from build123d import *

# Parameters (mm, degrees)
F2_DEPTH = 10


with BuildPart() as f2:
    # F1 (on Front) → F2 (new body)
    with BuildSketch(Plane.XZ):
        with BuildLine():
            Line((3.4480698746, 29.0000970366), (1.2642837874, 35))
            Line((1.2642837874, 35), (-1.2642837874, 35))
            Line((-1.2642837874, 35), (-3.4480698746, 29.0000970366))
            ThreePointArc((-3.4480698746, 29.0000970366), (-3.8654423248, 28.4561666695), (-4.5193194622, 28.25))
            Line((-4.5193194622, 28.25), (-4.7123889804, 28.25))
            Line((-4.7123889804, 28.25), (-4.7123889804, 0))
            Line((-4.7123889804, 0), (4.7123889804, 0))
            Line((4.7123889804, 0), (4.7123889804, 28.25))
            Line((4.7123889804, 28.25), (4.5193194622, 28.25))
            ThreePointArc((4.5193194622, 28.25), (3.8654423248, 28.4561666695), (3.4480698746, 29.0000970366))
        make_face()
        with BuildLine():
            Line((4.9054584985, 28.25), (4.7123889804, 28.25))
            Line((4.7123889804, 28.25), (4.7123889804, 0))
            Line((4.7123889804, 0), (14.1371669412, 0))
            Line((14.1371669412, 0), (14.1371669412, 28.25))
            Line((14.1371669412, 28.25), (13.944097423, 28.25))
            ThreePointArc((13.944097423, 28.25), (13.2902202856, 28.4561666695), (12.8728478353, 29.0000970366))
            Line((12.8728478353, 29.0000970366), (10.6890617482, 35))
            Line((10.6890617482, 35), (8.1604941734, 35))
            Line((8.1604941734, 35), (5.9767080862, 29.0000970366))
            ThreePointArc((5.9767080862, 29.0000970366), (5.559335636, 28.4561666695), (4.9054584985, 28.25))
        make_face()
        with BuildLine():
            Line((14.1371669412, 28.25), (14.1371669412, 0))
            Line((14.1371669412, 0), (23.5619449019, 0))
            Line((23.5619449019, 0), (23.5619449019, 28.25))
            Line((23.5619449019, 28.25), (23.3688753838, 28.25))
            ThreePointArc((23.3688753838, 28.25), (22.7149982463, 28.4561666695), (22.2976257961, 29.0000970366))
            Line((22.2976257961, 29.0000970366), (20.1138397089, 35))
            Line((20.1138397089, 35), (17.5852721341, 35))
            Line((17.5852721341, 35), (15.401486047, 29.0000970366))
            ThreePointArc((15.401486047, 29.0000970366), (14.9841135967, 28.4561666695), (14.3302364593, 28.25))
            Line((14.3302364593, 28.25), (14.1371669412, 28.25))
        make_face()
        with BuildLine():
            Line((23.5619449019, 28.25), (23.5619449019, 0))
            Line((23.5619449019, 0), (32.9867228627, 0))
            Line((32.9867228627, 0), (32.9867228627, 28.25))
            Line((32.9867228627, 28.25), (32.7936533446, 28.25))
            ThreePointArc((32.7936533446, 28.25), (32.1397762071, 28.4561666695), (31.7224037569, 29.0000970366))
            Line((31.7224037569, 29.0000970366), (29.5386176697, 35))
            Line((29.5386176697, 35), (27.0100500949, 35))
            Line((27.0100500949, 35), (24.8262640078, 29.0000970366))
            ThreePointArc((24.8262640078, 29.0000970366), (24.4088915575, 28.4561666695), (23.7550144201, 28.25))
            Line((23.7550144201, 28.25), (23.5619449019, 28.25))
        make_face()
        with BuildLine():
            Line((32.9867228627, 28.25), (32.9867228627, 0))
            Line((32.9867228627, 0), (42.4115008235, 0))
            Line((42.4115008235, 0), (42.4115008235, 28.25))
            Line((42.4115008235, 28.25), (42.2184313053, 28.25))
            ThreePointArc((42.2184313053, 28.25), (41.5645541679, 28.4561666695), (41.1471817176, 29.0000970366))
            Line((41.1471817176, 29.0000970366), (38.9633956305, 35))
            Line((38.9633956305, 35), (36.4348280557, 35))
            Line((36.4348280557, 35), (34.2510419685, 29.0000970366))
            ThreePointArc((34.2510419685, 29.0000970366), (33.8336695183, 28.4561666695), (33.1797923808, 28.25))
            Line((33.1797923808, 28.25), (32.9867228627, 28.25))
        make_face()
        with BuildLine():
            Line((42.4115008235, 28.25), (42.4115008235, 0))
            Line((42.4115008235, 0), (51.8362787842, 0))
            Line((51.8362787842, 0), (51.8362787842, 28.25))
            Line((51.8362787842, 28.25), (51.6432092661, 28.25))
            ThreePointArc((51.6432092661, 28.25), (50.9893321287, 28.4561666695), (50.5719596784, 29.0000970366))
            Line((50.5719596784, 29.0000970366), (48.3881735912, 35))
            Line((48.3881735912, 35), (45.8596060165, 35))
            Line((45.8596060165, 35), (43.6758199293, 29.0000970366))
            ThreePointArc((43.6758199293, 29.0000970366), (43.258447479, 28.4561666695), (42.6045703416, 28.25))
            Line((42.6045703416, 28.25), (42.4115008235, 28.25))
        make_face()
        with BuildLine():
            Line((51.8362787842, 28.25), (51.8362787842, 0))
            Line((51.8362787842, 0), (61.261056745, 0))
            Line((61.261056745, 0), (61.261056745, 28.25))
            Line((61.261056745, 28.25), (61.0679872269, 28.25))
            ThreePointArc((61.0679872269, 28.25), (60.4141100894, 28.4561666695), (59.9967376392, 29.0000970366))
            Line((59.9967376392, 29.0000970366), (57.812951552, 35))
            Line((57.812951552, 35), (55.2843839772, 35))
            Line((55.2843839772, 35), (53.1005978901, 29.0000970366))
            ThreePointArc((53.1005978901, 29.0000970366), (52.6832254398, 28.4561666695), (52.0293483024, 28.25))
            Line((52.0293483024, 28.25), (51.8362787842, 28.25))
        make_face()
        with BuildLine():
            Line((61.261056745, 28.25), (61.261056745, 0))
            Line((61.261056745, 0), (70.6858347058, 0))
            Line((70.6858347058, 0), (70.6858347058, 28.25))
            Line((70.6858347058, 28.25), (70.4927651876, 28.25))
            ThreePointArc((70.4927651876, 28.25), (69.8388880502, 28.4561666695), (69.4215155999, 29.0000970366))
            Line((69.4215155999, 29.0000970366), (67.2377295128, 35))
            Line((67.2377295128, 35), (64.709161938, 35))
            Line((64.709161938, 35), (62.5253758508, 29.0000970366))
            ThreePointArc((62.5253758508, 29.0000970366), (62.1080034006, 28.4561666695), (61.4541262631, 28.25))
            Line((61.4541262631, 28.25), (61.261056745, 28.25))
        make_face()
        with BuildLine():
            Line((70.6858347058, 28.25), (70.6858347058, 0))
            Line((70.6858347058, 0), (80.1106126665, 0))
            Line((80.1106126665, 0), (80.1106126665, 28.25))
            Line((80.1106126665, 28.25), (79.9175431484, 28.25))
            ThreePointArc((79.9175431484, 28.25), (79.263666011, 28.4561666695), (78.8462935607, 29.0000970366))
            Line((78.8462935607, 29.0000970366), (76.6625074735, 35))
            Line((76.6625074735, 35), (74.1339398988, 35))
            Line((74.1339398988, 35), (71.9501538116, 29.0000970366))
            ThreePointArc((71.9501538116, 29.0000970366), (71.5327813613, 28.4561666695), (70.8789042239, 28.25))
            Line((70.8789042239, 28.25), (70.6858347058, 28.25))
        make_face()
        with BuildLine():
            Line((80.1106126665, 28.25), (80.1106126665, 0))
            Line((80.1106126665, 0), (89.5353906273, 0))
            Line((89.5353906273, 0), (89.5353906273, 28.25))
            Line((89.5353906273, 28.25), (89.3423211092, 28.25))
            ThreePointArc((89.3423211092, 28.25), (88.6884439717, 28.4561666695), (88.2710715215, 29.0000970366))
            Line((88.2710715215, 29.0000970366), (86.0872854343, 35))
            Line((86.0872854343, 35), (83.5587178595, 35))
            Line((83.5587178595, 35), (81.3749317724, 29.0000970366))
            ThreePointArc((81.3749317724, 29.0000970366), (80.9575593221, 28.4561666695), (80.3036821847, 28.25))
            Line((80.3036821847, 28.25), (80.1106126665, 28.25))
        make_face()
        with BuildLine():
            Line((89.5353906273, 28.25), (89.5353906273, 0))
            Line((89.5353906273, 0), (98.9601685881, 0))
            Line((98.9601685881, 0), (98.9601685881, 28.25))
            Line((98.9601685881, 28.25), (98.7670990699, 28.25))
            ThreePointArc((98.7670990699, 28.25), (98.1132219325, 28.4561666695), (97.6958494822, 29.0000970366))
            Line((97.6958494822, 29.0000970366), (95.5120633951, 35))
            Line((95.5120633951, 35), (92.9834958203, 35))
            Line((92.9834958203, 35), (90.7997097331, 29.0000970366))
            ThreePointArc((90.7997097331, 29.0000970366), (90.3823372829, 28.4561666695), (89.7284601454, 28.25))
            Line((89.7284601454, 28.25), (89.5353906273, 28.25))
        make_face()
        with BuildLine():
            Line((98.9601685881, 28.25), (98.9601685881, 0))
            Line((98.9601685881, 0), (108.3849465488, 0))
            Line((108.3849465488, 0), (108.3849465488, 28.25))
            Line((108.3849465488, 28.25), (108.1918770307, 28.25))
            ThreePointArc((108.1918770307, 28.25), (107.5379998933, 28.4561666695), (107.120627443, 29.0000970366))
            Line((107.120627443, 29.0000970366), (104.9368413559, 35))
            Line((104.9368413559, 35), (102.4082737811, 35))
            Line((102.4082737811, 35), (100.2244876939, 29.0000970366))
            ThreePointArc((100.2244876939, 29.0000970366), (99.8071152437, 28.4561666695), (99.1532381062, 28.25))
            Line((99.1532381062, 28.25), (98.9601685881, 28.25))
        make_face()
    extrude(amount=F2_DEPTH)


solid = f2.part
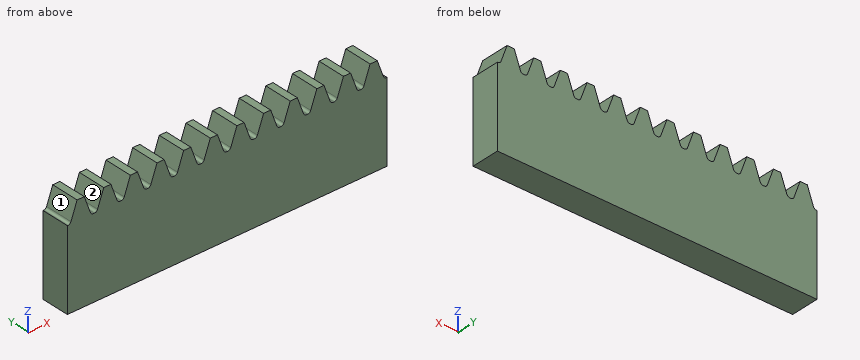
Part model, mm, in its own coordinate system. Face numbers are marked on the shaded views. A direction names the side the tool comes from. Round coordinates to 2 decimals unless told otherwise and drop trailing zeros. Answer as a JSON object with one key per item and string values.
Item 1: Wall check: L1, parallel to Z at x = 71, y = -7; L2, parallel to Z at x = 81, y = -9. Give the ranges that are in metal, low to high.
Output:
{"L1": "0 to 28.26", "L2": "0 to 28.49"}
Item 2: Band-saw the part on A-A on z = 30. State how many separate pieces and enclosed holes the cut face has, plus the area to 3 significant figures.
Output:
{"separate pieces": "12", "enclosed holes": "0", "area": "740 mm2"}
Item 3: Tool access for the marked faces 1 and 2: list every direction of +Z, -Z, +X, -X, +Y, -Y with a clear straight run to the whole face (end or side of a thin tool).
Output:
{"face 1": "+Z, -X, +Y, -Y", "face 2": "+Z, +Y, -Y"}
